Geometry check sheet. Reference: the model listing, model coordinates, mm. A direction names the side the tool comes from. Round coordinates to 2 decimals unless told otherwise and drop trailing zeros. Order: outer loops, then holes, each group sorted by start corner. A loop starts at its lowest first (then second) coordinate and runs counter-clockwise, first axis right, second up. Notation, with made-up numbers: (88.25, 26.5) - (126.25, 26.5) arc R23 cw to (126.25, 44.5) - close; hole circle Ø7 at (33, 85). An arc over 180 degrees is marked (long way). One line per question, with ' | ' between items. Start each with the question number.
Q1. Sectioned sample at B-B, the plane x = 27.5. Enter the section's corners in (y, z), then the cut area to 3 significant figures.
Q2. Gauge pin test, flat end, axial feed: P1, Ø5, axis at y = 8.5, z = 1368.5, coming from the +X side. Record the tip position at first contact, or that the pin passes through.
Q3. Sectioned sample at A-A, the plane z = 883.5. Enter the section's corners in (x, y), then the cut area to 3 significant figures.
Q4. Material ranges on line 1 along Y through (x, z) = (40.5, 1178); line 2 along Y through (x, z) = (10, 1660); line 3 along X through (y, z) = (-18, 724), recorded low to high.
Q5. Mould release check, pull along Y, two halves, no side actions. Record for faces 3 (the face through (3, 0, 0)), 4 (the face through (-1.43, -1, 847)), 5 (the face through (25.81, 32.71, 848.4)): +Y half, -Y half, draft (parallel to the pull), parting line (faces both ways), or undercut.
Q6. Tool access check on faces 1 (the face through (3, 0, 1720)), 2 (the face through (4.07, 0, 848)). Record the directions out of +Z, -Z, +X, -X, +Y, -Y that give a thin tool (end or side, any length) a straight path to the whole face; none if there is none.
Q7. Sectioned sample at C-C, the plane y = 4.5. Enter the section's corners in (x, z).
Autodesk Inventor part; units mm, degrees
ref_plane "Начальная плоскость" through (0, 0, -40) normal (0, 0, 1) x (1, 0, 0)
ref_plane "Конечная плоскость" through (0, 0, 1760) normal (0, 0, 1) x (1, 0, 0)
ref_plane "РабПлоскость4" through (21.07, -40, -40) normal (0, 0.7071, -0.7071) x (1, 0, 0)
ref_plane "Начальная плоскость" through (0, 0, -40) normal (0, 0, 1) x (1, 0, 0)
ref_plane "Конечная плоскость" through (0, 0, 1760) normal (0, 0, 1) x (1, 0, 0)
sketch "Эскиз" plane through (0, 0, 0) normal (0, 0, 1) x (1, 0, 0)
  line L0 (-1.43, 0) -> (-1.43, 40)
  line L1 (-1.43, 40) -> (43.57, 40)
  line L2 (43.57, 40) -> (43.57, 38.1774)
  line L3 (39.9881, 34.1993) -> (11.2338, 31.1771)
  line L4 (4.07, 23.221) -> (4.07, 0)
  line L5 (4.07, 0) -> (-1.43, 0) construction
  line L6 (23.82, 40) -> (23.82, 32.5) construction
  line L7 (43.57, 34.5758) -> (43.57, 32.5) construction
  line L8 (43.57, 32.5) -> (23.82, 32.5) construction
  line L9 (0, 15) -> (0, -27) construction
  line L10 (-5.539, 0) -> (16.0067, 0) construction
  line L11 (-1.43, 0) -> (-1.43, -40)
  line L12 (-1.43, -40) -> (43.57, -40)
  line L13 (43.57, -40) -> (43.57, -38.1774)
  line L14 (39.9881, -34.1993) -> (11.2338, -31.1771)
  line L15 (4.07, -23.221) -> (4.07, 0)
  arc A0 (11.2338, 31.1771) -> (4.07, 23.221) centre (12.07, 23.221) ccw
  arc A1 (4.07, -23.221) -> (11.2338, -31.1771) centre (12.07, -23.221) ccw
  arc A2 (39.9881, 34.1993) -> (43.57, 38.1774) centre (39.57, 38.1774) ccw
  arc A3 (43.57, -38.1774) -> (39.9881, -34.1993) centre (39.57, -38.1774) ccw
  line L16 (0, 56) -> (0, -56) construction
  line L17 (-15.5135, 0) -> (54.308, 0) construction
  point P0 (4.07, 30.4242)
  point P1 (43.57, -34.5758)
  point P2 (4.07, -30.4242)
  point P3 (23.82, -40)
  point P4 (23.82, -32.5)
  dimension "d0" = 5.5
  dimension "d1" = 40
  dimension "d2" = 45
  dimension "d3" = 7.5
  dimension "d4" = 19.75
  dimension "d5" = 2.0758
  dimension "d23" = 8
  dimension "d24" = 4
  dimension "d25" = 1.43
extrude "Тело" add sketch "Эскиз" along normal up to surface (1800 mm away) from surface at -40
sketch "Sketch3" plane through (0, 0, 0) normal (0, 0, 1) x (1, 0, 0)
  line L0 (0, 0) -> (10, 0)
ref_plane "Work Plane3" through (0, 0, 0) normal (0, -1, 0) x (1, 0, 0)
sketch "Sketch4" plane through (0, 0, 0) normal (0, -1, 0) x (1, 0, 0)
  line L0 (-2, -40) -> (12, -40)
  line L1 (-2, 1760) -> (12, 1760)
  dimension "d29" = 1800
ref_plane "РабПлоскость4" through (21.07, -40, -40) normal (0, 0.7071, -0.7071) x (1, 0, 0)
split "Разделение1" plane through (21.07, -40, -40) removes the side toward (0, 0.7071, -0.7071)
ref_plane "РабПлоскость5" through (21.07, -40, 1760) normal (0, 0.7071, 0.7071) x (1, 0, 0)
split "Разделение2" plane through (21.07, -40, 1760) removes the side toward (0, 0.7071, 0.7071)
equation "\"d0\" = G_T"
equation "\"d1\" = 0.5 * G_H"
equation "\"d2\" = G_W"
equation "\"d3\" = G_T1"
equation "\"d4\" = G_C"
equation "\"d23\" = G_IR"
equation "\"d24\" = G_ER"
equation "\"d25\" = ex"
equation "\"d6\" = G_L"
equation "\"G_W\" = 45"
equation "\"G_T\" = 5.5"
equation "\"G_T1\" = 7.5"
equation "\"G_NG\" = 0.105104"
equation "\"G_ER\" = 4"
equation "\"G_IR\" = 8"
equation "\"G_C\" = 19.75"
equation "\"G_L\" = d29"
equation "\"ex\" = 1.43"
properties part number "ISO 657/11 - CH 80 x 8 - 1800" material "Сталь, мягкая"
Determined:
1) outline: (-40, -40) - (-32.89, -32.89) - (-32.89, 1752.89) - (-40, 1760) - close; (32.89, 32.89) - (40, 40) - (40, 1680) - (32.89, 1687.11) - close | area: 24,500 mm2
2) P1: stops at x = 4.07
3) outline: (-1.43, -40) - (43.57, -40) - (43.57, -38.18) arc R4 ccw to (39.99, -34.2) - (11.23, -31.18) arc R8 cw to (4.07, -23.22) - (4.07, 23.22) arc R8 cw to (11.23, 31.18) - (39.99, 34.2) arc R4 ccw to (43.57, 38.18) - (43.57, 40) - (-1.43, 40) - close | area: 1,050 mm2
4) line 1: y = -40 to -34.29, 34.29 to 40 | line 2: y = -40 to -30.95, 30.95 to 40 | line 3: x = -1.43 to 4.07
5) face 3: +Y half | face 4: draft | face 5: undercut
6) face 1: +Z, +X, -X, +Y | face 2: +Z, -Z, +X
7) outline: (-1.43, 4.5) - (4.07, 4.5) - (4.07, 1715.5) - (-1.43, 1715.5) - close
